Verification items for the finished model (mm, model axes). Round coordinates to 2 decimals unless told otherwise and drop trailing zeros. Write each loop counter-clockwise with the first axis right and the second up, starting at its lowest first coordinate (ties: lowest second). Pieces come first, ordered by that corner, then holes. Notation, with made-up numbers: M 46,72 L 79,72 A19 ccw 79,87 Z; hole C -26,40 d3. An arc over 180 degrees is marked long. Answer in a Markdown table with one row per item. Add a question column.
1. Go/stop test with a flat-tipped pin: pin 1 Ø8 at (x, z) = (0, -38.1) entering from -Y. Record where the tip stops, or that it passes through.
2. Material ranges on probe 1 along X at (y, z) = (2.1, -12.7); probe 2 along X at (y, z) = (0.95, 13); probe 3 along Z at (x, y) = (23.5, 0.2), recorded low to high.
3. Draft check along Z on faces 1 (the cylindrical face through (-37.376, 1.61, -50.036)), 2 (the cylindrical face through (26.167, 1.61, 15.135)), 3 (the flat face through (38.1, 2, 1)). Enter one of: pulls with the +Z half, pulls with the -Z half, needs draft (parallel to the pull), parting line crosses it, or undercut.
4. Sectioned sample at B-B on x = 0. Record the cut outline in (y, z) (3 decimals).
5. Sectioned sample at C-C on y = 2.65. Count the separate pieces of the cut face and the enclosed holes in it, plus the area to 3 significant figures.
6. Sectioned sample at A-A on z = 38.1. Record the cut outline in (x, y) (3 decimals), plus the area to 3 significant figures.
```python
from build123d import *

# Parameters (mm, degrees)
SKETCH1_W            = 76.2
SKETCH1_H            = 101.6
BOSS_EXTRUDE1_DEPTH  = 3.175
SKETCH2_R            = 2.5527
CUT_EXTRUDE1_DEPTH   = 3.175
LPATTERN1_COUNT      = 4
LPATTERN1_PITCH      = 25.4
LPATTERN1_COUNT_DIR2 = 3
LPATTERN1_PITCH_DIR2 = 25.4
FILLET1_R            = 2.54


with BuildPart() as part:
    # Sketch1 → Boss-Extrude1 (new body)
    with BuildSketch(Plane(origin=(0, 0, 0), x_dir=(1, 0, 0), z_dir=(0, 1, 0))):
        Rectangle(SKETCH1_W, SKETCH1_H)
    extrude(amount=BOSS_EXTRUDE1_DEPTH)

    # Sketch2 → Cut-Extrude1 (cut)
    with BuildSketch(Plane(origin=(0, 3.175, 0), x_dir=(1, 0, 0), z_dir=(0, 1, 0))):
        with Locations(Location((-25.4, -38.1, 0), (0, 0, 270))):
            Circle(SKETCH2_R)
    cut_extrude1 = extrude(amount=-CUT_EXTRUDE1_DEPTH, mode=Mode.SUBTRACT)

    # LPattern1: Cut-Extrude1 4 × 3
    with Locations(*[(j * LPATTERN1_PITCH_DIR2, 0, -i * LPATTERN1_PITCH) for i in range(LPATTERN1_COUNT) for j in range(LPATTERN1_COUNT_DIR2) if (i, j) != (0, 0)]):
        add(cut_extrude1, mode=Mode.SUBTRACT)

    # Fillet1
    fillet1_edges = [part.edges().sort_by_distance(p)[0] for p in [
        (38.1, 1.5875, 50.8),
        (-38.1, 1.5875, 50.8),
        (-38.1, 1.5875, -50.8),
        (38.1, 1.5875, -50.8),
    ]]
    fillet(fillet1_edges, radius=FILLET1_R)


solid = part.part
```
Geometry check:
| question | item | result |
|---|---|---|
| 1 | pin 1 | stops at y = 0 |
| 2 | probe 1 | x = -38.1 to -27.95, -22.85 to -2.55, 2.55 to 22.85, 27.95 to 38.1 |
| 2 | probe 2 | x = -38.1 to -27.94, -22.86 to -2.54, 2.54 to 22.86, 27.94 to 38.1 |
| 2 | probe 3 | z = -50.8 to -39.8, -36.4 to -14.4, -11 to 11, 14.4 to 36.4, 39.8 to 50.8 |
| 3 | face 1 | pulls with the -Z half |
| 3 | face 2 | undercut |
| 3 | face 3 | needs draft |
| 4 | outline | M 0,-50.8 L 3.175,-50.8 L 3.175,-40.653 L 0,-40.653 Z; M 0,-35.547 L 3.175,-35.547 L 3.175,-15.253 L 0,-15.253 Z; M 0,-10.147 L 3.175,-10.147 L 3.175,10.147 L 0,10.147 Z; M 0,15.253 L 3.175,15.253 L 3.175,35.547 L 0,35.547 Z; M 0,40.653 L 3.175,40.653 L 3.175,50.8 L 0,50.8 Z |
| 5 | separate pieces | 1 |
| 5 | enclosed holes | 12 |
| 5 | area | 7,490 mm2 |
| 6 | outline | M -38.1,0 L -27.953,0 L -27.953,3.175 L -38.1,3.175 Z; M -22.847,0 L -2.553,0 L -2.553,3.175 L -22.847,3.175 Z; M 2.553,0 L 22.847,0 L 22.847,3.175 L 2.553,3.175 Z; M 27.953,0 L 38.1,0 L 38.1,3.175 L 27.953,3.175 Z |
| 6 | area | 193 mm2 |
